Autodesk Inventor part; units mm, degrees
ref_plane "YZ Plane" through (0, 0, 0) normal (1, 0, 0) x (0, 1, 0)
ref_plane "XZ Plane" through (0, 0, 0) normal (0, 1, 0) x (-1, 0, 0)
ref_plane "XY Plane" through (0, 0, 0) normal (0, 0, 1) x (1, 0, 0)
sketch "Sketch1" plane through (0, 0, 0) normal (0, 0, 1) x (1, 0, 0)
  circle A0 centre (0, 0) radius 11.25
  dimension "d0" = 22.5
extrude "Extrusion1" add sketch "Sketch1" along normal blind 25
sketch "Sketch2" plane through (0, 0, 0) normal (0, 0, -1) x (-1, 0, 0)
  line L0 (7.6788, 0) -> (3.8394, -6.65)
  line L1 (3.8394, -6.65) -> (-3.8394, -6.65)
  line L2 (-3.8394, -6.65) -> (-7.6788, 0)
  line L3 (-7.6788, 0) -> (-3.8394, 6.65)
  line L4 (-3.8394, 6.65) -> (3.8394, 6.65)
  line L5 (3.8394, 6.65) -> (7.6788, 0)
  point P0 (0, 0)
  point P1 (0, 0)
  dimension "d3" = 13.3
extrude "Extrusion2" cut sketch "Sketch2" against normal blind 30
sketch "Sketch3" plane through (0, 0, 25) normal (0, 0, 1) x (1, 0, 0)
  line L0 (3.8394, 6.65) -> (7.6788, 0)
  line L1 (7.6788, 0) -> (3.8394, -6.65)
  line L2 (3.8394, -6.65) -> (-3.8394, -6.65)
  line L3 (-3.8394, -6.65) -> (-7.6788, 0)
  line L4 (-7.6788, 0) -> (-3.8394, 6.65)
  line L5 (-3.8394, 6.65) -> (3.8394, 6.65)
  circle A0 centre (0, 0) radius 11.25
extrude "Extrusion3" add sketch "Sketch3" along normal blind 10
properties part number "tubo"
The listing builds one solid part. Answer for the finished solid, in the listing's coordinates (mm). A direction names the side the tool comes from. Give positions to 0.01 mm unless a question says otherwise; leave off trailing zeros. Loops run counter-clockwise (first coordinate to the right, second up) from the corner with the lowest first, then second, coordinate; pieces in that order, holes last. Notation, with made-up numbers: M 81.25,-26 L 96.25,-26 A19 ccw 96.25,-4 Z; hole C -7.75,67.5 d1. An arc over 180 degrees is marked long. One line per item, written item: value.
1. For a pull along Y with two mould halves and no side action, classify faces 3 (the face through (5.19, 9.98, 17.26)), 4 (the face through (-5, -5, 35)), 5 (the face through (-5.732, -3.372, 17.255)) as pulls with the +Y half, pulls with the -Y half, needs draft (parallel to the pull), parting line crosses it, or undercut.
Found:
face 3: parting line crosses it
face 4: needs draft
face 5: undercut
2. Section B-B on z = 14.5 is taken. Determine the outline of the cut face in (x, y).
Found:
outline: C 0,0 d22.5; hole M -7.68,0 L -3.84,-6.65 L 3.84,-6.65 L 7.68,0 L 3.84,6.65 L -3.84,6.65 Z
3. Section D-D on x = -8.75 is taken. Determine the outline of the cut face in (y, z), plus the area to 3 significant figures.
Found:
outline: M -7.07,0 L 7.07,0 L 7.07,35 L -7.07,35 Z
area: 495 mm^2
4. Each of these flat-tipped pins is pushed along its axis until it touches: P1, Ø2, axis at x = -4.5, z = 25, coming from the -Y side; P2, Ø4, axis at x = 3, z = 30.5, coming from the -Y side; P3, Ø2.5, axis at x = 1.5, z = 13, coming from the +Y side. Where does it stop, or does it pass through?
Found:
P1: y = -10.69
P2: y = -11.21
P3: y = 11.25
5. Find the intervals of material crossed by probe 1 along X at (y, z) = (3.5, 8); probe 2 along X at (y, z) = (3.75, 15.5); probe 3 along Y at (x, z) = (0.75, 6.5), in increasing order.
Found:
probe 1: -10.69 to -5.66, 5.66 to 10.69
probe 2: -10.61 to -5.51, 5.51 to 10.61
probe 3: -11.22 to -6.65, 6.65 to 11.22
6. For faces 1 (the face through (5.732, 3.372, 17.255)), 2 (the face through (-5, -5, 0)), determine the directions among +Z, -Z, +X, -X, +Y, -Y from which every point of the face is accessible in a straight line to the end or side of a thin tool.
Found:
face 1: +Z, -Z
face 2: -Z, +X, -X, +Y, -Y
7. Section A-A on x = 0 is taken. Determine the outline of the cut face in (y, z).
Found:
outline: M -11.25,0 L -6.65,0 L -6.65,35 L -11.25,35 Z; M 6.65,0 L 11.25,0 L 11.25,35 L 6.65,35 Z
8. Section C-C on y = -4 is taken. Determine the outline of the cut face in (x, z).
Found:
outline: M -10.51,0 L -5.37,0 L -5.37,35 L -10.51,35 Z; M 5.37,0 L 10.51,0 L 10.51,35 L 5.37,35 Z
